Check sheet for the modelled part. Datum: model origin and axes. Units: mm. Face numbers are marked on the shaded views. A direction names the side the tool comes from. Coordinates: 2 decimals unless noted, no trailing zeros. Loops run counter-clockwise (first coordinate to the right, second up) from the corner with the lowest first, then second, coordinate; pieces in that order, holes last. Notation, with made-up numbers: M 7,41 L 62,41 A25 ccw 62,72 Z; hole C 11,34.25 d3. An arc over 180 degrees is marked long. Return JSON: item names as keys, results as strings.
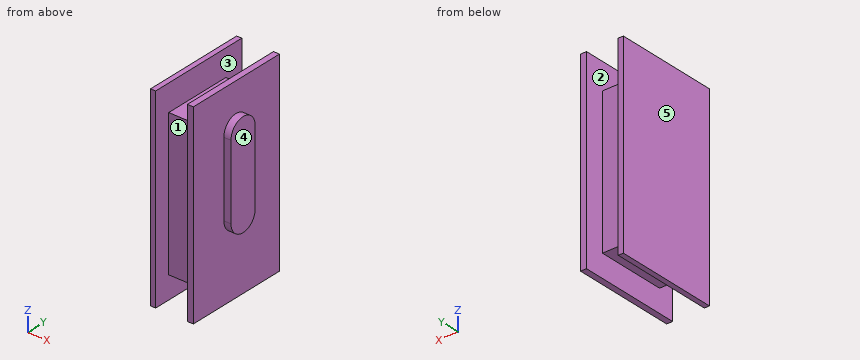
Autodesk Inventor part; units mm, degrees
ref_plane "YZ Plane" through (0, 0, 0) normal (1, 0, 0) x (0, 1, 0)
ref_plane "XZ Plane" through (0, 0, 0) normal (0, 1, 0) x (-1, 0, 0)
ref_plane "XY Plane" through (0, 0, 0) normal (0, 0, 1) x (1, 0, 0)
sketch "Sketch1" plane through (0, 0, 0) normal (1, 0, 0) x (0, 1, 0)
  line L0 (0, 0) -> (36.957, 0)
  line L1 (36.957, 0) -> (36.957, -69.088)
  line L2 (36.957, -69.088) -> (0, -69.088)
  line L3 (0, -69.088) -> (0, 0)
  dimension "d0" = 69.088
  dimension "d1" = 36.957
extrude "Extrusion1" add sketch "Sketch1" along normal blind 15.24
sketch "Sketch2" plane through (15.24, 0, 0) normal (1, 0, 0) x (0, 0, -1)
  line L0 (15.6183, 18.2767) -> (42.2027, 18.2767) construction
  line L1 (15.6183, 13.0907) -> (42.2027, 13.0907)
  line L2 (42.2027, 23.4628) -> (15.6183, 23.4628)
  arc A0 (15.6183, 23.4628) -> (15.6183, 13.0907) centre (15.6183, 18.2767) ccw
  arc A1 (42.2027, 13.0907) -> (42.2027, 23.4628) centre (42.2027, 18.2767) ccw
  point P0 (0, 0)
  point P1 (28.9105, 18.2767)
extrude "Extrusion2" add sketch "Sketch2" along normal blind 2.54
sketch "Sketch3" plane through (0, 0, -69.088) normal (0, 0, -1) x (-1, 0, 0)
  line L0 (-1.8203, -2.1906) -> (-13.1197, -2.1906)
  line L1 (-13.1197, -2.1906) -> (-13.1197, 2.4256)
  line L2 (-13.1197, 2.4256) -> (-1.8203, 2.4256)
  line L3 (-1.8203, 2.4256) -> (-1.8203, -2.1906)
  line L4 (-13.1197, 39.0109) -> (-1.8203, 39.0109)
  line L5 (-1.8203, 39.0109) -> (-1.8203, 33.2923)
  line L6 (-1.8203, 33.2923) -> (-13.1197, 33.2923)
  line L7 (-13.1197, 33.2923) -> (-13.1197, 39.0109)
  point P0 (0, 0)
extrude "Extrusion3" cut sketch "Sketch3" against normal blind 136.525
sketch "Sketch4" plane through (1.8203, 33.2923, -69.088) normal (0, 1, 0) x (1, 0, 0)
  line L0 (11.2994, 0) -> (11.2994, -69.088)
  line L1 (0, 0) -> (0, -69.088)
  line L2 (11.2994, 0) -> (0, 0)
  line L3 (0, 0) -> (0, -4.865)
  line L4 (0, -4.865) -> (11.2994, -4.865)
  line L5 (11.2994, -4.865) -> (11.2994, 0)
  line L6 (11.2994, -69.088) -> (13.4197, -69.088)
  line L7 (11.2994, -69.088) -> (0, -69.088)
  line L8 (0, -69.088) -> (0, -62.856)
  line L9 (0, -62.856) -> (11.2994, -62.856)
  line L10 (11.2994, -62.856) -> (11.2994, -69.088)
  point P0 (-1.8203, -69.088)
extrude "Extrusion4" cut sketch "Sketch4" against normal blind 136.525 contours L0 L4 L1 L2 | L0 L7 L1 L9
offset faces "Size1" outward -3.175 faces at (9.3532, 2.4256, -25.5623) (9.3532, 23.0034, -6.232) (5.5868, 33.2923, -44.8927) (5.5868, 23.0034, -64.223)
scale "Scale1" factors (0.7, 0.7, 0.7) then translate (0, 5.5436, -10.3632) bodies 1
properties part number "co2sensor"
1) Section check C-C on z = -24.5. Record the cut outline in (x, y).
Answers:
{"outline": "M 0,5.54 L 1.27,5.54 L 1.27,9.46 L 9.18,9.46 L 9.18,5.54 L 10.67,5.54 L 10.67,14.71 L 12.45,14.71 L 12.45,21.97 L 10.67,21.97 L 10.67,31.41 L 9.18,31.41 L 9.18,26.63 L 1.27,26.63 L 1.27,31.41 L 0,31.41 Z"}
2) Section check D-D on x = 11.75. Record the cut outline in (y, z).
Answers:
{"outline": "M 14.71,-39.91 A3.63 ccw 21.97,-39.91 L 21.97,-21.3 A3.63 ccw 14.71,-21.3 Z"}
3) Draft check along X on the marked faces 3, 4 and 5. Enter one of: +X half, -X half, draft (parallel to the pull), parting line (faces both ways), or undercut.
Answers:
{"face 3": "undercut", "face 4": "+X half", "face 5": "-X half"}
4) Go/stop test with flat-tipped pins: pin 1 Ø4 at (x, y) = (4, 25.5) entering from +Z; pin 2 Ø4 at (x, z) = (6, -25) entering from -Y; pin 3 Ø1 at (x, y) = (3.5, 28.5) entering from -Z; pin 4 Ø0.5 at (x, z) = (11.5, -33.5) entering from -Y. Record where each tip stops, or that it passes through.
Answers:
{"pin 1": "z = -16.95", "pin 2": "y = 9.46", "pin 3": "through", "pin 4": "y = 14.71"}
5) Set-up check for the marked faces 1 and 2: record each of +Z, -Z, +X, -X, +Y, -Y from which the full face is reachable in a straight line by a thin tool's end or side.
Answers:
{"face 1": "+Z, -Z, -Y", "face 2": "none"}
6) Section check A-A on y = 7.75. Record the cut outline in (x, z).
Answers:
{"outline": "M 0,-58.72 L 1.27,-58.72 L 1.27,-10.36 L 0,-10.36 Z; M 9.18,-58.72 L 10.67,-58.72 L 10.67,-10.36 L 9.18,-10.36 Z"}
7) Section check B-B on z = -14. Record the cut outline in (x, y).
Answers:
{"outline": "M 0,5.54 L 1.27,5.54 L 1.27,31.41 L 0,31.41 Z; M 9.18,5.54 L 10.67,5.54 L 10.67,31.41 L 9.18,31.41 Z"}
8) Scan lines: line 1 along X through (y, z) = (16.5, -55); line 2 along Y through (x, z) = (7.25, -33); line 3 along Z through (x, y) = (5, 16.5). Record each from-to range of solid material in increasing order. Write a range as [from, to].
Answers:
{"line 1": "[0, 1.27], [9.18, 10.67]", "line 2": "[9.46, 26.63]", "line 3": "[-53.1, -16.95]"}
